from build123d import *

# Parameters (mm, degrees)
CROQUIS1_R              = 2.5
SALIENTE_EXTRUIR1_DEPTH = 3


with BuildPart() as part:
    # Croquis1 → Saliente-Extruir1 (new body)
    with BuildSketch(Plane(origin=(0, 0, 0), x_dir=(1, 0, 0), z_dir=(0, 1, 0))):
        with BuildLine():
            Line((-60, 55), (60, 55))
            ThreePointArc((60, 55), (67.071067812, 52.071067812), (70, 45))
            Line((70, 45), (70, -35))
            Line((70, -35), (75, -35))
            ThreePointArc((75, -35), (78.535533906, -36.464466094), (80, -40))
            Line((80, -40), (80, -45))
            ThreePointArc((80, -45), (77.071067812, -52.071067812), (70, -55))
            Line((70, -55), (-70, -55))
            ThreePointArc((-70, -55), (-77.071067812, -52.071067812), (-80, -45))
            Line((-80, -45), (-80, -40))
            ThreePointArc((-80, -40), (-78.535533906, -36.464466094), (-75, -35))
            Line((-75, -35), (-70, -35))
            Line((-70, -35), (-70, 45))
            ThreePointArc((-70, 45), (-67.071067812, 52.071067812), (-60, 55))
        make_face()
        with Locations(Location((-60, 45, 0), (0, 0, 270))):
            Circle(CROQUIS1_R, mode=Mode.SUBTRACT)
        with Locations(Location((60, 45, 0), (0, 0, 270))):
            Circle(CROQUIS1_R, mode=Mode.SUBTRACT)
        with Locations(Location((-70, -45, 0), (0, 0, 270))):
            Circle(CROQUIS1_R, mode=Mode.SUBTRACT)
        with Locations(Location((70, -45, 0), (0, 0, 270))):
            Circle(CROQUIS1_R, mode=Mode.SUBTRACT)
    extrude(amount=SALIENTE_EXTRUIR1_DEPTH)


solid = part.part
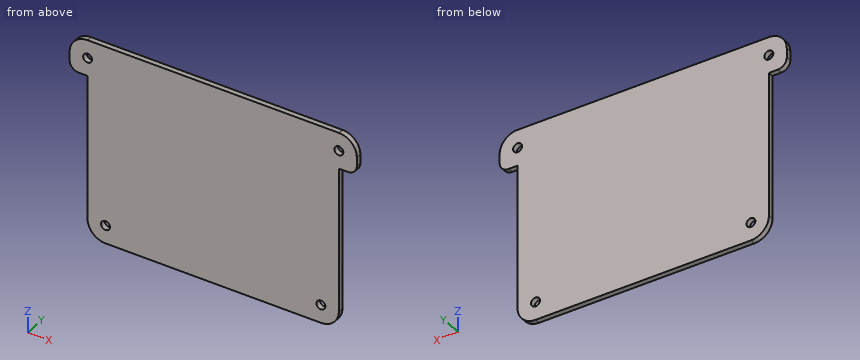
Input: part model. Units: mm. Frame: model coordinates. Coordinates: 2 decimals unless noted, no trailing zeros. Loops run counter-clockwise (first coordinate to the right, second up) from the corner with the lowest first, then second, coordinate; pieces in that order, holes last. Notation, with made-up numbers: (59, 67.25) - (80, 67.25) arc R36 cw to (80, 101.25) - close; hole circle Ø4 at (54, -8.75). An arc over 180 degrees is marked (long way). Answer in a Markdown table with one row per item. Add a question column.
Item 1: Contact query for flat-ended pins moving along their axis: P1, Ø0.9, axis at y = 1, z = -5, coming from the +X side; P2, Ø1.5, axis at y = 1, z = -20, coming from the -X side; P3, Ø4.5, axis at x = 60, z = -45, coming from the -Y side. Output: stop coordinate, or through.
Item 2: Line query: line 1 along X through (y, z) = (1.7, -45); line 2 along X through (y, z) = (2.45, 45); line 3 along X through (y, z) = (2.75, 33). Output: solid intervals per line, ascending. Write a range as [from, to].
Item 3: Section query A-A on y = 0.8. Return the cut outline in (x, z).
Item 4: Section query B-B on z = 32. Return the cut outline in (x, y), then the cut area to 3 significant figures.
Recorded:
| question | item | result |
|---|---|---|
| 1 | P1 | x = 70 |
| 1 | P2 | x = -70 |
| 1 | P3 | through |
| 2 | line 1 | [-70, -62.5], [-57.5, 57.5], [62.5, 70] |
| 2 | line 2 | [-80, -72.5], [-67.5, 67.5], [72.5, 80] |
| 2 | line 3 | [-70, 70] |
| 3 | outline | (-80, 40) arc R5 ccw to (-75, 35) - (-70, 35) - (-70, -45) arc R10 ccw to (-60, -55) - (60, -55) arc R10 ccw to (70, -45) - (70, 35) - (75, 35) arc R5 ccw to (80, 40) - (80, 45) arc R10 ccw to (70, 55) - (-70, 55) arc R10 ccw to (-80, 45) - close; hole circle Ø5 at (-70, 45); hole circle Ø5 at (-60, -45); hole circle Ø5 at (60, -45); hole circle Ø5 at (70, 45) |
| 4 | outline | (-70, 0) - (70, 0) - (70, 3) - (-70, 3) - close |
| 4 | area | 420 mm^2 |
